Build history of the part. All positions in model axes, mm. A direction names the side the tool comes from. Give positions to 0.01 mm unless a question says otherwise; leave off trailing zeros. Order: outer loops, then holes, each group sorted by start corner. A loop starts at its lowest first (then second) coordinate and runs counter-clockwise, first axis right, second up. Notation, with made-up numbers: (-17, 30.25) - (18, 30.25) arc R14 ccw to (18, 38.25) - close; hole circle Ø6 at (53, 52.5). An arc over 180 degrees is marked (long way). Use a Markdown table: item, result.
from build123d import *

# Parameters (mm, degrees)
SKETCH1_W           = 24
SKETCH1_H           = 30
BOSS_EXTRUDE1_DEPTH = 11
SKETCH2_R           = 1.65
CUT_EXTRUDE1_DEPTH  = 30
SKETCH3_R           = 10.2
CUT_EXTRUDE2_DEPTH  = 24
SKETCH5_W           = 40
SKETCH5_H           = 40
BOSS_EXTRUDE3_DEPTH = 5
SKETCH8_W           = 40
SKETCH8_H           = 40
SKETCH8_W_2         = 28
SKETCH8_H_2         = 28
BOSS_EXTRUDE4_DEPTH = 10
SKETCH9_R           = 1.65
CUT_EXTRUDE3_DEPTH  = 15
FILLET3_R           = 4
SKETCH10_W          = 24
SKETCH10_H          = 30
BOSS_EXTRUDE5_DEPTH = 5
FILLET6_R           = 8


with BuildPart() as part:
    # Sketch1 → Boss-Extrude1 (new body, symmetric)
    with BuildSketch(Plane(origin=(0, 0, 0), x_dir=(1, 0, 0), z_dir=(0, 1, 0))):
        Rectangle(SKETCH1_W, SKETCH1_H)
    extrude(amount=BOSS_EXTRUDE1_DEPTH, both=True)

    # Sketch2 → Cut-Extrude1 (cut)
    with BuildSketch(Plane(origin=(0, 0, -15), x_dir=(-1, 0, 0), z_dir=(0, 0, -1))):
        with Locations((4, 0)):
            Circle(SKETCH2_R)
        with Locations((-4, 0)):
            Circle(SKETCH2_R)
    extrude(amount=-CUT_EXTRUDE1_DEPTH, mode=Mode.SUBTRACT)

    # Sketch3 → Cut-Extrude2 (cut)
    with BuildSketch(Plane.ZY.offset(12)):
        Circle(SKETCH3_R)
    extrude(amount=-CUT_EXTRUDE2_DEPTH, mode=Mode.SUBTRACT)

    # Sketch5 → Boss-Extrude3 (add)
    with BuildSketch(Plane(origin=(0, 16, 0), x_dir=(1, 0, 0), z_dir=(0, 1, 0))):
        Rectangle(SKETCH5_W, SKETCH5_H)
    extrude(amount=-BOSS_EXTRUDE3_DEPTH)

    # Sketch8 → Boss-Extrude4 (add)
    with BuildSketch(Plane(origin=(0, 16, 0), x_dir=(1, 0, 0), z_dir=(0, 1, 0))):
        Rectangle(SKETCH8_W, SKETCH8_H)
        Rectangle(SKETCH8_W_2, SKETCH8_H_2, mode=Mode.SUBTRACT)
    extrude(amount=BOSS_EXTRUDE4_DEPTH)

    # Sketch9 → Cut-Extrude3 (cut)
    with BuildSketch(Plane(origin=(0, 26, 0), x_dir=(1, 0, 0), z_dir=(0, 1, 0))):
        with Locations((-16, 16)):
            Circle(SKETCH9_R)
        with Locations((16, 16)):
            Circle(SKETCH9_R)
        with Locations((16, -16)):
            Circle(SKETCH9_R)
        with Locations((-16, -16)):
            Circle(SKETCH9_R)
    extrude(amount=-CUT_EXTRUDE3_DEPTH, mode=Mode.SUBTRACT)

    # Fillet3
    fillet3_edges = [part.edges().sort_by_distance(p)[0] for p in [
        (20, 18.5, 20),
        (20, 18.5, -20),
        (-20, 18.5, -20),
        (-20, 18.5, 20),
        (-14, 21, 14),
        (-14, 21, -14),
        (14, 21, -14),
        (14, 21, 14),
    ]]
    fillet(fillet3_edges, radius=FILLET3_R)

    # Sketch10 → Boss-Extrude5 (add)
    with BuildSketch(Plane.XZ.offset(11)):
        Rectangle(SKETCH10_W, SKETCH10_H)
    extrude(amount=BOSS_EXTRUDE5_DEPTH)

    # Fillet6
    fillet6_edges = [part.edges().sort_by_distance(p)[0] for p in [
        (0, -16, 15),
        (0, -16, -15),
    ]]
    fillet(fillet6_edges, radius=FILLET6_R)


solid = part.part
1) Slice it at B-B (x = -7.5). Write the cut outline in (y, z).
Computed:
| item | result |
|---|---|
| outline | (-16, -7) arc R8 ccw to (-8, -15) - (11, -15) - (11, -20) - (26, -20) - (26, -14) - (16, -14) - (16, 14) - (26, 14) - (26, 20) - (11, 20) - (11, 15) - (-8, 15) arc R8 ccw to (-16, 7) - close; hole circle Ø20.4 at (0, 0) |
2) Wall check: line 1 (Z direction, x = 16, y = 19.75); line 2 (X direction, y = 0, z = 12). Give the ranges that are in metal, low to high. Write a range as from..to.
Computed:
| item | result |
|---|---|
| line 1 | z = -20..-17.65, -14.35..14.35, 17.65..20 |
| line 2 | x = -12..-5.65, -2.35..2.35, 5.65..12 |
3) Pin check, flat tips, straight feed: P1, Ø9.5, axis at x = 0.5, y = 4.5, coming from the +Z side; P2, Ø4, axis at x = 16, z = 16, coming from the -Y side; P3, Ø22.5, axis at x = -0.5, z = 2, coming from the +Y side. Stop position of each tip, or through.
Computed:
| item | result |
|---|---|
| P1 | stops at z = 15 |
| P2 | stops at y = 11 |
| P3 | stops at y = 16 |
4) Tool access for faces 5 (the flat face through (0, 2, 15)), 6 (the flat face through (12, -11, 0)), 7 (the cylindrical face through (12.859, 21.07, -12.797)): list every direction of +Z, -Z, +X, -X, +Y, -Y with a clear straight run to the whole face (end or side of a thin tool).
Computed:
| item | result |
|---|---|
| face 5 | +Z, +X, -X, -Y |
| face 6 | +Z, -Z, +X, -Y |
| face 7 | +Y |
5) Slice it at C-C (y = 19.5). Write the cut outline in (x, z).
Computed:
| item | result |
|---|---|
| outline | (-20, -16) arc R4 ccw to (-16, -20) - (16, -20) arc R4 ccw to (20, -16) - (20, 16) arc R4 ccw to (16, 20) - (-16, 20) arc R4 ccw to (-20, 16) - close; hole circle Ø3.3 at (-16, -16); hole circle Ø3.3 at (-16, 16); hole (-14, -10) arc R4 ccw to (-10, -14) - (10, -14) arc R4 ccw to (14, -10) - (14, 10) arc R4 ccw to (10, 14) - (-10, 14) arc R4 ccw to (-14, 10) - close; hole circle Ø3.3 at (16, -16); hole circle Ø3.3 at (16, 16) |
6) Slice it at D-D (y = 3). Write the cut outline in (x, z).
Computed:
| item | result |
|---|---|
| outline | (-12, -15) - (12, -15) - (12, -9.75) - (-12, -9.75) - close; (-12, 9.75) - (12, 9.75) - (12, 15) - (-12, 15) - close |
7) Slice it at A-A (z = 5). Write the cut outline in (x, y), and give its area (3 significant figures).
Computed:
| item | result |
|---|---|
| outline | (-20, 11) - (-12, 11) - (-12, 8.89) - (12, 8.89) - (12, 11) - (20, 11) - (20, 26) - (14, 26) - (14, 16) - (-14, 16) - (-14, 26) - (-20, 26) - close; (-12, -16) - (12, -16) - (12, -8.89) - (-12, -8.89) - close |
| area | 541 mm² |
8) Two-plate mould, pull along X, no slides. Class faces 1 (the cylindrical face through (-2.35, 0.07, -12.57)), 2 (the cylindrical face through (18.797, 18.395, -18.859)), 3 (the cylindrical face through (-14.476, 18.605, -15.368)), 4 (the flat face through (-18, 26, 0)): +X half, -X half, draft (parallel to the pull), parting line (faces both ways), or undercut.
Computed:
| item | result |
|---|---|
| face 1 | undercut |
| face 2 | +X half |
| face 3 | undercut |
| face 4 | draft |
